Geometry: final body of the model. Coordinates: model frame, mm. Coordinates: 2 decimals unless noted, no trailing zeros. Order: outer loops, then holes, each group sorted by start corner. A loop starts at its lowest first (then second) coordinate and runs counter-clockwise, first axis right, second up. Notation, with made-up numbers: M -25,-34.5 L -8,-34.5 A6 cw -8,-29.5 Z; hole C 29.5,68 d3. An arc over 180 degrees is marked long. Use CSV: the item, a comma, the result in double quotes. Start each with the question number.
1. Section query A-A on x = 1. Return the cut outline in (y, z) (1 decimal).
2. Material intervals for line 1 (Z direction, x = 3.75, y = 3); line 2 (Z direction, x = -4.5, y = 17); line 3 (X direction, y = -22, z = 7), sorted ascending.
3. First-contact query: P1, Ø4, axis at y = 19, z = 7.18, coming from the -X side; P2, Ø2, axis at x = -2, y = 2.5, coming from the -Z side; P3, Ø6, axis at x = -3.5, z = 20, coming from the +Y side. Flat tips, straight axial feed; report the tip coordinate or a pass-through.
4. Pull-direction query (Z, two-part tool) for faces 1 (the flat face through (6.35, 5, 12)), 2 (the cylindrical face through (0.09, -1.82, 8.3)), 3 (the cylindrical face through (-5.364, -7.629, -11.527)); classes: pulls with the +Z half, pulls with the -Z half, needs draft (parallel to the pull), parting line crosses it, or undercut.
from build123d import *

# Parameters (mm, degrees)
SKETCH3_R          = 4.7625
CUT_EXTRUDE1_DEPTH = 48.519048812
CUT_EXTRUDE2_REACH = 49.519
SKETCH4_R          = 2.38125


with BuildPart() as part:
    # Sketch2 → Revolve1 (revolve)
    with BuildSketch(Plane(origin=(0, 0, 0), x_dir=(1, 0, 0), z_dir=(0, 1, 0))):
        with BuildLine():
            Line((-4.35, -12.7), (4.35, -12.7))
            Line((4.35, -12.7), (4.35, 12.441505181))
            ThreePointArc((4.35, 12.441505181), (0, 8.342326358), (-4.35, 12.441505181))
            Line((-4.35, 12.441505181), (-4.35, -12.7))
        make_face()
        Polygon((-6.35, -12.7), (-4.35, -12.7), (-4.35, 12.441505181), (-4.35, 12.7), (-6.35, 12.7), align=None)
        with BuildLine():
            Line((4.35, -12.7), (6.35, -12.7))
            Line((6.35, -12.7), (6.35, 12.7))
            Line((6.35, 12.7), (4.357673642, 12.7))
            ThreePointArc((4.357673642, 12.7), (4.355754809, 12.570695653), (4.35, 12.441505181))
            Line((4.35, 12.441505181), (4.35, -12.7))
        make_face()
    revolve(axis=Axis((6.35, 0, 12.7), (-1, 0, 0)))

    # Sketch3 → Cut-Extrude1 (cut, through all)
    with BuildSketch(Plane(origin=(6.35, 0, 0), x_dir=(0, 0, -1), z_dir=(1, 0, 0))):
        with Locations((-12.7, 0)):
            Circle(SKETCH3_R)
    extrude(amount=-CUT_EXTRUDE1_DEPTH, mode=Mode.SUBTRACT)

    # Sketch4 → Cut-Extrude2 (cut, up to next)
    with BuildSketch(Plane(origin=(6.35, 0, 0), x_dir=(0, 0, -1), z_dir=(1, 0, 0)), mode=Mode.PRIVATE) as cut_extrude2_sk1:
        with Locations((-7.184338108, 19)):
            Circle(SKETCH4_R)
    cut_extrude2_tool1 = extrude(cut_extrude2_sk1.sketch, amount=-CUT_EXTRUDE2_REACH, mode=Mode.PRIVATE) & part.part
    add(cut_extrude2_tool1.solids().sort_by_distance((6.35, 19, 7.184338))[0], mode=Mode.SUBTRACT)


solid = part.part
Results list:
1,outline,"M 19.7,4.9 A2.4 cw long 20.8,8.8 A21.2 ccw long Z; hole C 0,12.7 d9.5"
2,line 1,"z = -10.29 to 9, 16.4 to 35.69"
2,line 2,"z = -6.17 to 5.89, 8.48 to 31.57"
2,line 3,"x = -6.35 to -3.44, 3.44 to 6.35"
3,P1,"passes through"
3,P2,"stops at z = -9.4"
3,P3,"stops at y = 25.01"
4,face 1,"needs draft"
4,face 2,"undercut"
4,face 3,"parting line crosses it"
